Autodesk Inventor part; units mm, degrees
ref_plane "YZ Plane" through (0, 0, 0) normal (1, 0, 0) x (0, 1, 0)
ref_plane "XZ Plane" through (0, 0, 0) normal (0, 1, 0) x (-1, 0, 0)
ref_plane "XY Plane" through (0, 0, 0) normal (0, 0, 1) x (1, 0, 0)
sketch "スケッチ1" plane through (0, 0, 0) normal (0, 0, 1) x (1, 0, 0)
  circle A0 centre (-34.3, -20) radius 1.6
  circle A1 centre (-34.3, 0) radius 1.6
  circle A2 centre (-34.3, -40) radius 1.6
  circle A3 centre (34.3, -20) radius 1.6
  circle A4 centre (34.3, 0) radius 1.6
  circle A5 centre (34.3, -40) radius 1.6
  circle A6 centre (0, 0) radius 1.6
  circle A7 centre (0, 0) radius 50 construction
  circle A8 centre (0, -60.2) radius 10 construction
  circle A9 centre (0, -60.2) radius 12.55
  circle A10 centre (-12.3744, -47.8256) radius 2.15
  circle A11 centre (-12.3744, -72.5744) radius 2.15
  circle A12 centre (12.3744, -72.5744) radius 2.15
  circle A13 centre (12.3744, -47.8256) radius 2.15
  line L0 (12.3744, -47.8256) -> (-12.3744, -47.8256) construction
  line L1 (-12.3744, -47.8256) -> (-12.3744, -72.5744) construction
  line L2 (-12.3744, -72.5744) -> (12.3744, -72.5744) construction
  line L3 (12.3744, -72.5744) -> (12.3744, -47.8256) construction
  line L4 (12.3744, -47.8256) -> (-12.3744, -72.5744) construction
  line L5 (-12.3744, -47.8256) -> (12.3744, -72.5744) construction
  line L6 (-41.8, 7.5) -> (41.8, 7.5)
  line L7 (41.8, 7.5) -> (41.8, -42.5528)
  line L8 (41.8, -42.5528) -> (16.3361, -75.6247)
  line L9 (-41.8, 7.5) -> (-41.8, -42.5528)
  line L10 (-41.8, -42.5528) -> (-16.3361, -75.6247)
  arc A14 (-16.3361, -75.6247) -> (-12.3744, -77.5744) centre (-12.3744, -72.5744) ccw
  arc A15 (12.3744, -77.5744) -> (16.3361, -75.6247) centre (12.3744, -72.5744) ccw
  line L11 (-12.3744, -77.5744) -> (12.3744, -77.5744)
  circle A16 centre (20, -60.2) radius 1.6
  circle A17 centre (-20, -60.2) radius 1.6
  dimension "d0" = 3.2
  dimension "d1" = 3.2
  dimension "d2" = 3.2
  dimension "d3" = 20
  dimension "d4" = 20
  dimension "d5" = 3.2
  dimension "d6" = 3.2
  dimension "d7" = 3.2
  dimension "d8" = 20
  dimension "d9" = 20
  dimension "d10" = 68.6
  dimension "d11" = 34.3
  dimension "d12" = 3.2
  dimension "d13" = 100
  dimension "d14" = 20
  dimension "d15" = 60.2
  dimension "d16" = 25.1
  dimension "d17" = 4.3
  dimension "d18" = 4.3
  dimension "d19" = 4.3
  dimension "d20" = 4.3
  dimension "d21" = 35
  dimension "d22" = 5
  dimension "d23" = 7.5
  dimension "d24" = 7.5
  dimension "d25" = 7.5
  dimension "d26" = 7.5
  dimension "d27" = 7.5
  dimension "d31" = 3.2
  dimension "d32" = 3.2
  dimension "d33" = 40
  dimension "d34" = 20
extrude "押し出し1" add sketch "スケッチ1" along normal blind 3
fillet "フィレット1" radius 2 4 edges at (-41.8, 7.5, 1.5) (41.8, 7.5, 1.5) (41.8, -42.5528, 1.5) (-41.8, -42.5528, 1.5)
properties part number "関節4_側板" material "アルミニウム 6061"
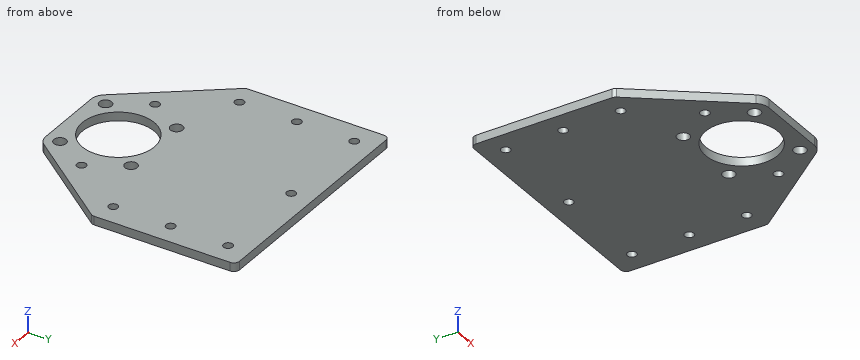
For this review, take the finished solid that the model builds, in its own axes (mm). Round coordinates to 2 decimals unless told otherwise and drop trailing zeros. Loops run counter-clockwise (first coordinate to the right, second up) from the corner with the lowest first, then second, coordinate; pieces in that order, holes last. Notation, with made-up numbers: (15.25, 7) - (33.25, 7) arc R10 ccw to (33.25, 19) - close; hole circle Ø4 at (-24.5, 34.5). An arc over 180 degrees is marked (long way). Use one line per item in the form item = value.
Item 1: Consider section D-D on x = -34.5. Write out the cut boundary in (y, z), then the cut area to 3 significant figures.
Answers:
outline = (-52.03, 0) - (-41.59, 0) - (-41.59, 3) - (-52.03, 3) - close; (-38.41, 0) - (-21.59, 0) - (-21.59, 3) - (-38.41, 3) - close; (-18.41, 0) - (-1.59, 0) - (-1.59, 3) - (-18.41, 3) - close; (1.59, 0) - (7.5, 0) - (7.5, 3) - (1.59, 3) - close
area = 150 mm^2
Item 2: Consider section C-C on y = -20. Write out the cut boundary in (x, z).
Answers:
outline = (-41.8, 0) - (-35.9, 0) - (-35.9, 3) - (-41.8, 3) - close; (-32.7, 0) - (32.7, 0) - (32.7, 3) - (-32.7, 3) - close; (35.9, 0) - (41.8, 0) - (41.8, 3) - (35.9, 3) - close
Item 3: Consider section B-B on x = 0. Write out the cut boundary in (y, z), then the cut area to 3 significant figures.
Answers:
outline = (-77.57, 0) - (-72.75, 0) - (-72.75, 3) - (-77.57, 3) - close; (-47.65, 0) - (-1.6, 0) - (-1.6, 3) - (-47.65, 3) - close; (1.6, 0) - (7.5, 0) - (7.5, 3) - (1.6, 3) - close
area = 170 mm^2
Item 4: Consider section A-A on y = 0. Write out the cut boundary in (x, z), then the cut area to 3 significant figures.
Answers:
outline = (-41.8, 0) - (-35.9, 0) - (-35.9, 3) - (-41.8, 3) - close; (-32.7, 0) - (-1.6, 0) - (-1.6, 3) - (-32.7, 3) - close; (1.6, 0) - (32.7, 0) - (32.7, 3) - (1.6, 3) - close; (35.9, 0) - (41.8, 0) - (41.8, 3) - (35.9, 3) - close
area = 222 mm^2
Item 5: Clearance check with a flat-ended pin moving along its axis: P1, Ø1.5, axis at y = -58, z = 1.5, coming from the +X side. State where the tip first meets the part, or that it passes through.
Answers:
P1 = 30.48
Item 6: For line 1 (Y direction, x = 0, z = 0.95); line 2 (Y direction, x = 10.5, z = 1.45); line 3 (Y direction, x = 34.3, z = 2.05), list the stretches that pass through material, from the lowest coordinate up.
Answers:
line_1 = -77.57 to -72.75, -47.65 to -1.6, 1.6 to 7.5
line_2 = -77.57 to -73.63, -71.52 to -67.07, -53.33 to -48.88, -46.77 to 7.5
line_3 = -52.29 to -41.6, -38.4 to -21.6, -18.4 to -1.6, 1.6 to 7.5
